Can you work these out from the model? Positions are in its coordinate system, mm. Coordinates: 2 decimals unless noted, no trailing zeros. Order: outer loops, then holes, each group sorted by start corner. A loop starts at its lowest first (then second) coordinate and runs counter-clockwise, first axis right, second up. Notation, with made-up numbers: (-2.75, 12) -> (11.25, 12) arc R27 ccw to (11.25, 46) -> close; hole circle Ø9 at (88, 44.5). An arc over 180 degrees is marked (long way). Answer as a JSON object with one key per item and string values. Group by question number.
(1) I want a section at A-A, the plane x = 0. List the corners of the cut face in (y, z) for me, plus the area to 3 significant figures.
(2) For pin 1 (5 mm diameter, centred on x = -28.99, y = -28.99, fed in from +Z); pin 2 (5 mm diameter, centred on y = -32.5, z = 2.5, fed in from -X); pin 3 (1.5 mm diameter, centred on x = 32, y = 14, fed in from +Z); pin 4 (1.5 mm diameter, centred on x = -29.5, z = 2.5, fed in from -Y), each with a flat end and sliding along its axis, tell me the tip position at first contact or that it passes through.
(3) I need wall thicknesses on line 1 (Y direction, x = -41, z = 5.45); line 2 (Y direction, x = 3, z = 1.5); line 3 (Z direction, x = -23.5, y = 25.5). Which ranges of each line are inside material? Lowest first, please.
(4) If we mould it in two halves opening along Y, with no side actions, what happens to faces 1 (the cylindrical face through (1.245, 37.998, 4.859)), 2 (the cylindrical face through (-4.036, -30.736, 7.479)), 3 (the conical face through (18.052, 43.008, 0.142))? For each: pulls with the +Y half, pulls with the -Y half, needs draft (parallel to the pull), parting line crosses it, or undercut.
(5) I want a section at C-C, the plane z = 7.5. List the corners of the cut face in (x, y) for me.
Solid Edge part; units mm, degrees
sketch "Sketch1" plane through (0, 0, 0) normal (0, 0, 1) x (1, 0, 0)
  circle A0 centre (0, 0) radius 47
extrude "Protrusion1" add sketch "Sketch1" along normal blind 6
sketch "Sketch2" plane through (0, 0, 6) normal (0, 0, 1) x (1, 0, 0)
  circle A0 centre (0, 0) radius 31
extrude "ProtrusiónExtruida_2" add sketch "Sketch2" along normal blind 3
sketch "Sketch3" plane through (0, 0, 9) normal (0, 0, 1) x (1, 0, 0)
  circle A0 centre (0, 0) radius 28
extrude "VaciadoExtruido_1" cut sketch "Sketch3" against normal blind 6
sketch "Sketch4" plane through (0, 0, 3) normal (0, 0, 1) x (1, 0, 0)
  circle A0 centre (0, 0) radius 23
extrude "Cutout1" cut sketch "Sketch4" against normal through all
chamfer "Chaflán_1" distance 0.5 angle 45 2 edges at (-47, 0, 0) (-47, 0, 6)
sketch "Sketch5" plane through (0, 0, 0) normal (1, 0, 0) x (0, 1, 0)
  line L0 (-37.75, 6) -> (-37.75, 3.75)
  line L1 (-37.75, 3.75) -> (-34, 0)
  dimension "D1" = 37.75
revolve "RevolvedCutout1" cut sketch "Sketch5" angle 360 about axis through (0, -41, 17.975) along (0, 0, -1) material side at (0, -37.8, 4.875)
pattern_circular "Pattern1" count 8 over 360 about axis through (0, 0, 0) along (0, 0, 1) of "RevolvedCutout1"
properties part number "1976-1100-003" material "Aluminio, 7075-T6"
Computed values:
{
 "1": {"outline": "(-47, 1) -> (-44.25, 3.75) -> (-44.25, 6) -> (-46.5, 6) -> (-47, 5.5) -> close; (-37.75, 3.75) -> (-34, 0) -> (-23, 0) -> (-23, 3) -> (-28, 3) -> (-28, 9) -> (-31, 9) -> (-31, 6) -> (-37.75, 6) -> close; (23, 0) -> (34, 0) -> (37.75, 3.75) -> (37.75, 6) -> (31, 6) -> (31, 9) -> (28, 9) -> (28, 3) -> (23, 3) -> close; (44.25, 3.75) -> (47, 1) -> (47, 5.5) -> (46.5, 6) -> (44.25, 6) -> close", "area": "171 mm2"},
 "2": {"pin 1": "passes through", "pin 2": "stops at x = -36.18", "pin 3": "stops at z = 6", "pin 4": "stops at y = -37.18"},
 "3": {"line 1": "y = -22.98 to -3.25, 3.25 to 22.98", "line 2": "y = -46.9 to -45.61, -36.39 to -22.8, 22.8 to 36.39, 45.61 to 46.9", "line 3": "z = 0.49 to 6"},
 "4": {"face 1": "undercut", "face 2": "parting line crosses it", "face 3": "pulls with the +Y half"},
 "5": {"outline": "circle Ø62 at (0, 0); hole circle Ø56 at (0, 0)"}
}
